Can you work these out from the drawing? Everything is in mm from the part's minimum corner. A direction names the side the tool comes from. Coordinates: 2 decimals unless noted, no trailing zeros. Write each loop counter-clockwise with the first axis right and the second up, starting at its lowest first coordinate (ties: lowest second). Pieces come first, ordered by that corner, then holes.
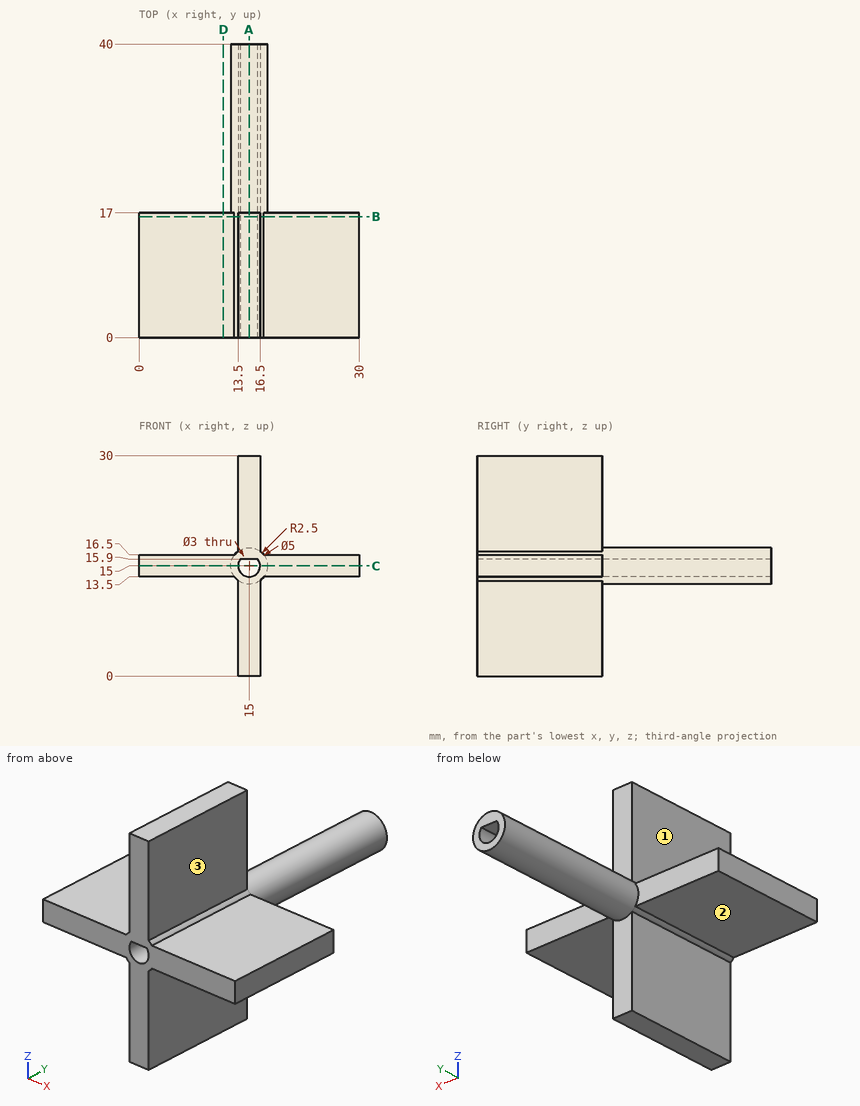
1. I want a section at A-A (x = 15). List the corners of the cut face in (y, z) for me, then the cut area to 3 significant figures.
2. I want a section at C-C (z = 15). List the corners of the cut face in (x, y) for me, then the cut area to 3 significant figures.
3. I want a section at B-B (y = 16.5). List the corners of the cut face in (x, z) for me.
4. If I drill on line 1 (X direction, y = 18.5, z = 15); line 2 (Z direction, x = 15, y = 9); line 3 (Z direction, x = 15, y = 27.5), over which ranges is the centre line in solid material (lowest first)?
5. For pin 1 Ø10 at (x, y) = (5, 18.5) entering from +Z; pin 2 Ø4 at (x, y) = (8, 6) entering from -Z; pin 3 Ø10.5 at (y, z) = (12.5, 9.5) entering from +X; pin 4 Ø3.5 at (x, z) = (14.5, 22.5) entering from +Y, each with a flat end and sliding along its axis, tell me the tip position at first contact or that it passes through.
6. I want a section at D-D (x = 11.5). List the corners of the cut face in (y, z) for me.
7. On a 3-axis mill with a long thin cutter (end or side, diameter ignored), from which of +Z, -Z, +X, -X, +Y, -Y can I reach the whole of each face in a straight line? I mean the marked faces 1, 2 and 3. Say none if no direction works.
Response values:
1. outline: (0, 0) - (17, 0) - (17, 12.5) - (40, 12.5) - (40, 13.5) - (0, 13.5) - close; (0, 15.9) - (40, 15.9) - (40, 17.5) - (17, 17.5) - (17, 30) - (0, 30) - close
1. area: 529 mm2
2. outline: (0, 0) - (13.5, 0) - (13.5, 40) - (12.5, 40) - (12.5, 17) - (0, 17) - close; (16.5, 0) - (30, 0) - (30, 17) - (17.5, 17) - (17.5, 40) - (16.5, 40) - close
2. area: 505 mm2
3. outline: (0, 13.5) - (13, 13.5) arc R2.5 ccw to (13.5, 13) - (13.5, 0) - (16.5, 0) - (16.5, 13) arc R2.5 ccw to (17, 13.5) - (30, 13.5) - (30, 16.5) - (17, 16.5) arc R2.5 ccw to (16.5, 17) - (16.5, 30) - (13.5, 30) - (13.5, 17) arc R2.5 ccw to (13, 16.5) - (0, 16.5) - close; hole (13.8, 15.9) arc R1.5 ccw (long way) to (16.2, 15.9) - close
4. line 1: x = 12.5 to 13.5, 16.5 to 17.5
4. line 2: z = 0 to 13.5, 15.9 to 30
4. line 3: z = 12.5 to 13.5, 15.9 to 17.5
5. pin 1: stops at z = 16.5
5. pin 2: stops at z = 13.5
5. pin 3: stops at x = 30
5. pin 4: stops at y = 17
6. outline: (0, 13.5) - (17, 13.5) - (17, 16.5) - (0, 16.5) - close
7. face 1: +Z, -X, +Y, -Y
7. face 2: -Z, -X, +Y, -Y
7. face 3: +Z, +X, +Y, -Y
